from build123d import *
from build123d.topology import SkipClean

# Parameters (mm, degrees)
BOSS_EXTRUDE1_DEPTH   = 7.62
BODY_MOVE_COPY5_ANGLE = 180
BOSS_EXTRUDE2_START   = -25.4
SKETCH4_R             = 9.5
BOSS_EXTRUDE2_DEPTH   = 146.05
LPATTERN2_COUNT       = 3
LPATTERN2_PITCH       = 146.05
BODY_MOVE_COPY6_ANGLE = 120
BODY_MOVE_COPY7_ANGLE = 120
BOSS_EXTRUDE3_START   = 24.94
SKETCH6_R             = 9.5
BOSS_EXTRUDE3_DEPTH   = 24.94


with BuildPart() as part:
    # Sketch2 → Boss-Extrude1 (new body)
    with BuildSketch(Plane.XY):
        with BuildLine():
            Line((-10.998522628, 6.35), (-5.499261314, 15.875))
            ThreePointArc((-5.499261314, 15.875), (0, 19.05), (5.499261314, 15.875))
            Line((5.499261314, 15.875), (10.998522628, 6.35))
            ThreePointArc((10.998522628, 6.35), (0, -12.7), (-10.998522628, 6.35))
        make_face()
    extrude(amount=BOSS_EXTRUDE1_DEPTH)


with BuildPart() as body_2:
    # Body-Move_Copy4: copy of part
    add(part.part.moved(Location((0, 0, 60.96))))


with BuildPart() as body_2_1:
    # Body-Move_Copy5: moved
    add(body_2.part.rotate(Axis((0, 0, 0), (0, 0, 1)), BODY_MOVE_COPY5_ANGLE))


with BuildPart() as part_1:
    add(part.part)

    add(body_2_1.part)  # Boss-Extrude2 merges body 2
    # Sketch4 → Boss-Extrude2 (add)
    with BuildSketch(Plane.XY.offset(BOSS_EXTRUDE2_START)):
        Circle(SKETCH4_R)
    extrude(amount=BOSS_EXTRUDE2_DEPTH)


with BuildPart() as lpattern2_1:
    # LPattern2: pattern copy
    add(part_1.part.moved(Location(Vector(0, 0, 1) * (1 * LPATTERN2_PITCH))))


with BuildPart() as lpattern2_2:
    # LPattern2: pattern copy
    add(part_1.part.moved(Location(Vector(0, 0, 1) * (2 * LPATTERN2_PITCH))))


with BuildPart() as lpattern2_1_1:
    # Body-Move_Copy6: moved
    add(lpattern2_1.part.rotate(Axis((0, 0, 0), (0, 0, 1)), BODY_MOVE_COPY6_ANGLE))


with BuildPart() as lpattern2_2_1:
    # Body-Move_Copy7: moved
    add(lpattern2_2.part.rotate(Axis((0, 0, 0), (0, 0, -1)), BODY_MOVE_COPY7_ANGLE))


with BuildPart() as part_2:
    with SkipClean():  # the faces are left unmerged after this step: merging them gives an invalid solid
        add(part_1.part)

        # Sketch6 → Boss-Extrude3 (add)
        with BuildSketch(Plane(origin=(0, 0, -25.4), x_dir=(-1, 0, 0), z_dir=(0, 0, -1)).offset(BOSS_EXTRUDE3_START)):
            with Locations(Location((0, 0, 0), (0, 0, 300))):
                Circle(SKETCH6_R)
        extrude(amount=-BOSS_EXTRUDE3_DEPTH)

    # Combine1: union LPattern2_1, LPattern2_2
    add(lpattern2_1_1.part)
    add(lpattern2_2_1.part)


solid = part_2.part
Source: CAD feature listing. Evaluate the final solid. Frame: model axes, mm. A direction names the side the tool comes from. Round coordinates to 2 decimals unless told otherwise and drop trailing zeros. Order: outer loops, then holes, each group sorted by start corner. A loop starts at its lowest first (then second) coordinate and runs counter-clockwise, first axis right, second up. Notation, with made-up numbers: (38, 66) - (83, 66) arc R22 cw to (83, 95) - close; hole circle Ø2 at (-16.75, 7). An arc over 180 degrees is marked (long way). Use a Markdown table: item, result. Add a question column.
1. Set-up query: faces 4 (the cylindrical face through (2.2, 9.24, 106.77)), 5 (the flat face through (-1, 10, 0)), 6 (the flat face through (-8.287, 11.046, 3.757)), 7 (the flat face through (8.2, 11.2, 3.8)), 8 (the flat face through (-5, -12.7, 150)). Return all of +Z, -Z, +X, -X, +Y, -Y with unobstructed straight access to the full face (end or side cutting, diameter ignored); none if empty.
2. Mould query, pull axis Z, two halves, no side actions, for faces 1 (the cylindrical face through (4.38, -8.43, 33.92)), 2 (the flat face through (-13.71, -1.65, 356.82)), 3 (the flat face through (0, 0, -50.34)). Classes: +Z half, -Z half, draft (parallel to the pull), parting line (faces both ways), or undercut.
3. Line query: probe 1 along Z at (x, y) = (8.5, -7.5); probe 2 along Z at (x, y) = (-11.5, 8.5); probe 3 along Y at (x, z) = (6.5, 295). Output: solid intervals per line, ascending.
4. Section query A-A (z = 132). Return the cut outline in (x, y).
5. First-contact query: pin 1 (8 mm diameter, centred on x = 14, y = -12.5, fed in from -Z); pin 2 (10 mm diameter, centred on x = 13.5, y = -12, fed in from +Z); pin 3 (1.5 mm diameter, centred on y = 3, z = 296, fed in from +X). Flat tips, straight axial feed; report the tip coordinate or a pass-through.
Derived:
| question | item | result |
|---|---|---|
| 1 | face 4 | none |
| 1 | face 5 | -Z |
| 1 | face 6 | -Z, -X, +Y |
| 1 | face 7 | -Z, +X, +Y |
| 1 | face 8 | +Z, +X, -X, -Y |
| 2 | face 1 | undercut |
| 2 | face 2 | draft |
| 2 | face 3 | -Z half |
| 3 | probe 1 | 0 to 7.62, 60.96 to 68.58, 146.05 to 153.67, 207.01 to 214.63, 292.1 to 299.72, 353.06 to 360.68 |
| 3 | probe 2 | 353.06 to 360.68 |
| 3 | probe 3 | -12.7 to 10.91 |
| 4 | outline | circle Ø19 at (0, 0) |
| 5 | pin 1 | z = 292.1 |
| 5 | pin 2 | z = 299.72 |
| 5 | pin 3 | x = 13.37 |
